Work out the finished part from the listing and answer in its coordinate system (mm). Face numbers are marked on the shaded views. A direction names the side the tool comes from. Round coordinates to 2 decimals unless told otherwise and drop trailing zeros. Loops run counter-clockwise (first coordinate to the right, second up) from the corner with the lowest first, then second, coordinate; pieces in that order, holes last.
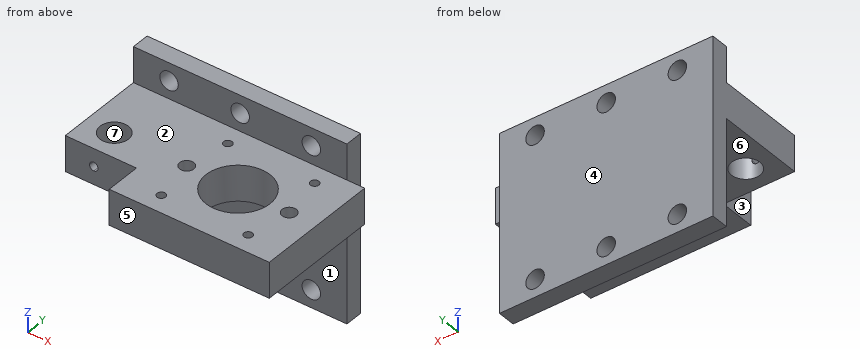
```python
from build123d import *

# Parameters (mm, degrees)
F0_W      = 76.2
F0_H      = 12.7
F0_R      = 3.302
F1_DEPTH  = 6.35
F0_H_2    = 38.1
F2_DEPTH  = 50.8
F4_R      = 1.524
F4_R_2    = 11.43
F4_R_3    = 5.08
F4_W      = 25.4
F4_H      = 12.7
F5_DEPTH  = 50.8
F6_DEPTH  = 25.4
F8_DEPTH  = 7.62
F9_W      = 44.45
F9_H      = 12.7
F10_DEPTH = 6.35
F12_DEPTH = 25.4


with BuildPart() as f1:
    # F0 (on Front) → F1 (new body)
    with BuildSketch(Plane.XZ):
        with Locations((-38.1, 6.35)):
            Rectangle(F0_W, F0_H)
        with Locations((-63.5, 6.35)):
            Circle(F0_R, mode=Mode.SUBTRACT)
        with Locations((-38.1, 6.35)):
            Circle(F0_R, mode=Mode.SUBTRACT)
        with Locations((-12.7, 6.35)):
            Circle(F0_R, mode=Mode.SUBTRACT)
    extrude(amount=F1_DEPTH)


with BuildPart() as f1b:
    # F0 (on Front) → F1, piece 2 (new body)
    with BuildSketch(Plane.XZ):
        with Locations((-38.1, -44.45)):
            Rectangle(F0_W, F0_H)
        with Locations((-63.5, -44.45)):
            Circle(F0_R, mode=Mode.SUBTRACT)
        with Locations((-38.1, -44.45)):
            Circle(F0_R, mode=Mode.SUBTRACT)
        with Locations((-12.7, -44.45)):
            Circle(F0_R, mode=Mode.SUBTRACT)
    extrude(amount=F1_DEPTH)


with BuildPart() as f2:
    # F0 (on Front) → F2 (new body)
    with BuildSketch(Plane.XZ):
        with Locations((-38.1, -19.05)):
            Rectangle(F0_W, F0_H_2)
    extrude(amount=F2_DEPTH)


with BuildPart() as f1_1:
    add(f1.part)

    # F3: union F1b, F2
    add(f1b.part)
    add(f2.part)

    # F4 (on face) → F5 (cut)
    with BuildSketch(Plane.XY):
        with Locations((-6.35, -44.069)):
            Circle(F4_R)
        with Locations((-6.35, -13.081)):
            Circle(F4_R)
        with Locations((-37.338, -13.081)):
            Circle(F4_R)
        with Locations((-37.338, -44.069)):
            Circle(F4_R)
        with Locations((-21.844, -28.575)):
            Circle(F4_R_2)
        with Locations((-66.04, -28.575)):
            Circle(F4_R_3)
        with Locations((-63.5, -44.45)):
            Rectangle(F4_W, F4_H)
    extrude(amount=-F5_DEPTH, mode=Mode.SUBTRACT)

    # F6 (cut): a face of the model
    f6_faces = [f1_1.faces().sort_by_distance(p)[0] for p in [
        (-36.7979159702, -26.5619005098, -38.1),
    ]]
    extrude(f6_faces, amount=-F6_DEPTH, mode=Mode.SUBTRACT)

    # F7 (on face) → F8 (cut)
    with BuildSketch(Plane.XZ.offset(38.1)):
        with BuildLine():
            ThreePointArc((-66.04, -7.874), (-64.9623692655, -7.4276307345), (-64.516, -6.35))
            ThreePointArc((-64.516, -6.35), (-64.9623692655, -5.2723692655), (-66.04, -4.826))
            ThreePointArc((-66.04, -4.826), (-67.1176307345, -5.2723692655), (-67.564, -6.35))
            ThreePointArc((-67.564, -6.35), (-67.1176307345, -7.4276307345), (-66.04, -7.874))
        make_face()
    extrude(amount=-F8_DEPTH, mode=Mode.SUBTRACT)

    # F9 (on face) → F10 (join)
    with BuildSketch(Plane.YZ):
        with Locations((-28.575, -6.35)):
            Rectangle(F9_W, F9_H)
    extrude(amount=F10_DEPTH)

    # F11 (on face) → F12 (cut)
    with BuildSketch(Plane(origin=(0, 0, -12.7), x_dir=(1, 0, 0), z_dir=(0, 0, -1))):
        with BuildLine():
            ThreePointArc((-1.016, 28.575), (-3.556, 31.115), (-6.096, 28.575))
            ThreePointArc((-6.096, 28.575), (-3.556, 26.035), (-1.016, 28.575))
        make_face()
        with BuildLine():
            ThreePointArc((-42.672, 28.575), (-40.132, 26.035), (-37.592, 28.575))
            ThreePointArc((-37.592, 28.575), (-40.132, 31.115), (-42.672, 28.575))
        make_face()
    extrude(amount=-F12_DEPTH, mode=Mode.SUBTRACT)


solid = f1_1.part
```
1. Consider probe 1 along X at (y, z) = (-5, 6); probe 2 along Z at (x, y) = (-63.5, -1.5); probe 3 along Y at (x, z) = (-66.04, -10) (3 decimals). Determine where each line is inside the solid, lowest interval first.
Answer key:
probe 1: x = -76.2 to -66.78, -60.22 to -41.38, -34.82 to -15.98, -9.42 to 0
probe 2: z = -50.8 to -47.75, -41.15 to 3.05, 9.65 to 12.7
probe 3: y = -38.1 to -33.655, -23.495 to 0
2. Find section A-A (z = 6.35). Write down the section's boundary in (x, y).
Answer key:
outline: (-76.2, -6.35) - (-66.8, -6.35) - (-66.8, 0) - (-76.2, 0) - close; (-60.2, -6.35) - (-41.4, -6.35) - (-41.4, 0) - (-60.2, 0) - close; (-34.8, -6.35) - (-16, -6.35) - (-16, 0) - (-34.8, 0) - close; (-9.4, -6.35) - (0, -6.35) - (0, 0) - (-9.4, 0) - close
3. Which of the six approach directions +Z, -Z, +X, -X, +Y, -Y give full straight-line access (tool end or side, diameter ignored) to the marked faces 1, 2, 3 and 4?
Answer key:
face 1: -Z, +X, -X, -Y
face 2: +Z, +X, -X, -Y
face 3: +Z, -Z, -X, -Y
face 4: +Z, -Z, +X, -X, +Y
4. Find section B-B (x = -63.5). Write down the section's boundary in (y, z).
Answer key:
outline: (-38.1, -12.7) - (-32.97, -12.7) - (-32.97, 0) - (-38.1, 0) - close; (-24.18, -12.7) - (-6.35, -12.7) - (-6.35, -41.15) - (0, -41.15) - (0, 3.05) - (-6.35, 3.05) - (-6.35, 0) - (-24.18, 0) - close; (-6.35, -50.8) - (0, -50.8) - (0, -47.75) - (-6.35, -47.75) - close; (-6.35, 9.65) - (0, 9.65) - (0, 12.7) - (-6.35, 12.7) - close
5. Given pin 1 (3 mm diameter, centred on y = -2, z = -14.5, fed in from +X); pin 2 (13.5 mm diameter, centred on x = -51.5, y = -31.5, fed in from +Z); pin 3 (14 mm diameter, centred on y = -42, z = -7, fed in from -X); pin 4 (4 mm diameter, centred on x = -60.5, z = -3.5, fed in from -Y), each flat-ended and moving along its own axis, determine where each tip first touches the part or whether it passes through.
Answer key:
pin 1: stops at x = 0
pin 2: stops at z = 0
pin 3: stops at x = -76.2
pin 4: stops at y = -38.1
6. Find section C-C (y = -27). Write down the section's boundary in (x, z), then the cut area to 3 significant figures.
Answer key:
outline: (-76.2, -12.7) - (-70.87, -12.7) - (-70.87, 0) - (-76.2, 0) - close; (-61.21, -12.7) - (-42.12, -12.7) - (-42.12, 0) - (-61.21, 0) - close; (-38.14, -12.7) - (-33.16, -12.7) - (-33.16, 0) - (-38.14, 0) - close; (-10.52, -12.7) - (-5.55, -12.7) - (-5.55, 0) - (-10.52, 0) - close; (-1.56, -12.7) - (6.35, -12.7) - (6.35, 0) - (-1.56, 0) - close
area: 537 mm2
7. Find section D-D (x = -32). Write down the section's boundary in (y, z).
Answer key:
outline: (-50.8, -12.7) - (-33.82, -12.7) - (-33.82, 0) - (-50.8, 0) - close; (-23.33, -12.7) - (-6.35, -12.7) - (-6.35, -50.8) - (0, -50.8) - (0, 12.7) - (-6.35, 12.7) - (-6.35, 0) - (-23.33, 0) - close
8. Determine the mould class of the marked faces 5, 6 and 7 for opening direction Y: +Y half, -Y half, draft (parallel to the pull), parting line (faces both ways), or undercut.
Answer key:
face 5: -Y half
face 6: draft
face 7: undercut
